The model under review builds one solid part; all positions refer to its coordinate system, in mm. A direction names the side the tool comes from. Round coordinates to 2 decimals unless told otherwise and drop trailing zeros. Write each loop counter-clockwise with the first axis right and the second up, starting at its lowest first coordinate (ties: lowest second). Pieces come first, ordered by that corner, then holes. Notation, with made-up numbers: M -30.75,-11 L -24.75,-11 A12 ccw -24.75,2 Z; hole C 39,10 d11. An arc over 180 degrees is marked long. Write item = value, one per line. Start each with the question number.
Item 1: To check wall thickness, follow line 1 along Y through (x, z) = (7, 0); line 2 along Z through (x, y) = (5.05, 2.5); line 3 along X through (y, z) = (6, 1.5). State the ranges of each line that lie inside material, in increasing order.
Item 2: Take a section at A-A, the plane y = 6.5. Give the boundary of the cut face in (x, z).
Item 3: The part is to be moulded in two halves that separate along X. For faces 1 (the flat face through (-1, 40, 0)), 2 (the cylindrical face through (-8.47, 43.25, 0.05)), 3 (the flat face through (-8.5, 14, 0)), say which applies: +X half, -X half, draft (parallel to the pull), parting line (faces both ways), or undercut.
Item 4: Take a section at D-D, the plane x = -1.75. Give the boundary of the cut face in (y, z), plus the area to 3 significant figures.
Item 5: Take a section at B-B, the plane x = -5. Give the boundary of the cut face in (y, z), plus the area to 3 significant figures.
Item 6: Tool access review of faces 4 (the flat face through (4.5, 43, 0)), 5 (the flat face through (-4, 4, 0)), 6 (the flat face through (-1, 24, 2.5)): name each direction out of +Z, -Z, +X, -X, +Y, -Y from which nothing blocks a thin tool from reaching the whole face with its end or side.
Item 7: For pin 1 Ø3 at (y, z) = (44.5, 0) entering from +X; pin 2 Ø1.5 at (y, z) = (2, -0.5) entering from -X; pin 3 Ø1.5 at (y, z) = (44.5, 0) entering from +X; pin 4 Ø1.5 at (x, z) = (-0.5, -0.5) entering from +Y, all flat-tipped, find the tip position at first contact; note any pin that passes through.
Item 8: Take a section at C-C, the plane z = -0.6. Give the number of separate pieces and of enclosed holes in the cut face, plus the area to 3 significant figures.
from build123d import *

# Parameters (mm, degrees)
F1_DEPTH      = 2.5
F2_R          = 1.25
F3_DEPTH      = 10.501
F3_DEPTH_BACK = 8.501


with BuildPart() as f1:
    # F0 (on Top) → F1 (new body, symmetric)
    with BuildSketch(Plane.XY):
        Polygon((-8.5, 27), (-8.5, 0), (-4, 0), (-4, 7), (4, 7), (4, 0), (8.5, 0), (8.5, 47), (4.5, 47), (4.5, 40), (-6.5, 40), (-6.5, 47), (-10.5, 47), (-10.5, 38), align=None)
    extrude(amount=F1_DEPTH, both=True)

    # F2 (on Right) → F3 (cut, two sides)
    with BuildSketch(Plane.YZ) as f3_sk:
        with Locations((2.5, 0)):
            Circle(F2_R)
        with BuildLine():
            ThreePointArc((2.5, -2.5), (0.732233047, -1.767766953), (0, 0))
            Line((0, 0), (0, -2.5))
            Line((0, -2.5), (2.5, -2.5))
        make_face()
        with BuildLine():
            ThreePointArc((0, 0), (0.732233047, 1.767766953), (2.5, 2.5))
            Line((2.5, 2.5), (0, 2.5))
            Line((0, 2.5), (0, 0))
        make_face()
        with Locations((44.5, 0)):
            Circle(F2_R)
        with BuildLine():
            ThreePointArc((44.5, 2.5), (46.267766953, 1.767766953), (47, 0))
            Line((47, 0), (47, 2.5))
            Line((47, 2.5), (44.5, 2.5))
        make_face()
        with BuildLine():
            ThreePointArc((47, 0), (46.267766953, -1.767766953), (44.5, -2.5))
            Line((44.5, -2.5), (47, -2.5))
            Line((47, -2.5), (47, 0))
        make_face()
    extrude(amount=-F3_DEPTH, mode=Mode.SUBTRACT)
    extrude(f3_sk.sketch, amount=F3_DEPTH_BACK, mode=Mode.SUBTRACT)


solid = f1.part
Response values:
q1.line_1 = 0 to 1.25, 3.75 to 43.25, 45.75 to 47
q1.line_2 = -2.5 to -1.25, 1.25 to 2.5
q1.line_3 = -8.5 to -4, 4 to 8.5
q2.outline = M -8.5,-2.5 L -4,-2.5 L -4,2.5 L -8.5,2.5 Z; M 4,-2.5 L 8.5,-2.5 L 8.5,2.5 L 4,2.5 Z
q3.face_1 = undercut
q3.face_2 = draft
q3.face_3 = -X half
q4.outline = M 7,-2.5 L 40,-2.5 L 40,2.5 L 7,2.5 Z
q4.area = 165 mm2
q5.outline = M 2.5,-2.5 L 40,-2.5 L 40,2.5 L 2.5,2.5 A2.5 ccw Z; hole C 2.5,0 d2.5
q5.area = 192 mm2
q6.face_4 = +Z, -Z, +Y
q6.face_5 = +Z, -Z, -Y
q6.face_6 = +Z, +X, -X, +Y, -Y
q7.pin_1 = 8.5
q7.pin_2 = -8.5
q7.pin_3 = through
q7.pin_4 = 40
q8.separate_pieces = 5
q8.enclosed_holes = 0
q8.area = 656 mm2
